Geometry check sheet. Reference: the model listing, model coordinates, mm. Give positions to 0.01 mm unless a question says otherwise; leave off trailing zeros. Order: outer loops, then holes, each group sorted by start corner. A loop starts at its lowest first (then second) coordinate and runs counter-clockwise, first axis right, second up. Notation, with made-up numbers: M 61,-26 L 69,-26 A23 cw 69,-14 Z; hole C -37,3 d4. An arc over 180 degrees is marked long. Answer as a JSON object with one key per item and string values. Group by question number.
from build123d import *

# Parameters (mm, degrees)
F1_DEPTH      = 15
F1_DEPTH_BACK = 15
F2_DEPTH      = 10
F2_DEPTH_BACK = 10
F3_DEPTH      = 5
F3_DEPTH_BACK = 5
F4_R          = 4.99999
F5_T8_DEPTH   = 31.3397459622
F5_S9_R       = 10
F5_T10_DEPTH  = 18
F5_T14_DEPTH  = 31.3397459622
F5_S15_R      = 10
F5_T16_DEPTH  = 18
F5_T20_DEPTH  = 31.3397459622
F5_S21_R      = 10
F5_T22_DEPTH  = 18
F5_T26_DEPTH  = 31.3397459622
F5_S27_R      = 10
F5_T28_DEPTH  = 18


# Not quite as in the source:
# - a fillet or chamfer that OpenCascade refuses, or shapes differently, is made with other operations: its cross-section is extruded or revolved along the edge and cut away or added
# - a fillet or chamfer is up to 0.001 mm smaller than in the source, because OpenCascade refuses the exact size


with BuildPart() as f1:
    # F0 (on Right) → F1 (new body, two sides)
    with BuildSketch(Plane.YZ) as f1_sk:
        with BuildLine():
            Line((-5, 16.4746102661), (5, 16.4746102661))
            ThreePointArc((5, 16.4746102661), (0, 21.4746102661), (-5, 16.4746102661))
        make_face()
        with BuildLine():
            ThreePointArc((-5, 16.4746102661), (0, 11.4746102661), (5, 16.4746102661))
            Line((5, 16.4746102661), (-5, 16.4746102661))
        make_face()
    extrude(amount=F1_DEPTH)
    extrude(f1_sk.sketch, amount=-F1_DEPTH_BACK)

    # F0 (on Right) → F2 (join, two sides)
    with BuildSketch(Plane.YZ) as f2_sk:
        with BuildLine():
            ThreePointArc((-5, 16.4746102661), (0, 21.4746102661), (5, 16.4746102661))
            Line((5, 16.4746102661), (5, 7.8143562283))
            ThreePointArc((5, 7.8143562283), (8.6602540378, 11.4746102661), (10, 16.4746102661))
            ThreePointArc((10, 16.4746102661), (-5, 25.1348643039), (-5, 7.8143562283))
            Line((-5, 7.8143562283), (-5, 16.4746102661))
        make_face()
        with BuildLine():
            Line((5, 7.8143562283), (5, 16.4746102661))
            ThreePointArc((5, 16.4746102661), (0, 11.4746102661), (-5, 16.4746102661))
            Line((-5, 16.4746102661), (-5, 7.8143562283))
            ThreePointArc((-5, 7.8143562283), (0, 6.4746102661), (5, 7.8143562283))
        make_face()
    extrude(amount=F2_DEPTH)
    extrude(f2_sk.sketch, amount=-F2_DEPTH_BACK)

    # F0 (on Right) → F3 (join, two sides)
    with BuildSketch(Plane.YZ) as f3_sk:
        with BuildLine():
            Line((5, 1.4746102661), (5, 7.8143562283))
            ThreePointArc((5, 7.8143562283), (0, 6.4746102661), (-5, 7.8143562283))
            Line((-5, 7.8143562283), (-5, 1.4746102661))
            Line((-5, 1.4746102661), (5, 1.4746102661))
        make_face()
    extrude(amount=F3_DEPTH)
    extrude(f3_sk.sketch, amount=-F3_DEPTH_BACK)

    # F4 (radius 5 in the source; OpenCascade refuses exactly that, so slightly less here)
    f4_edges = [f1.edges().sort_by_distance(p)[0] for p in [
        (15, 5, 16.47461),
        (-15, 5, 16.47461),
    ]]
    fillet(f4_edges, radius=F4_R)

    # F5: fillet of radius 5 on 8 edges, made by hand

    # F5_s1 → F5_t2 (revolve, cut)
    with BuildSketch(Plane.XY.offset(16.4746102661)):
        with BuildLine():
            ThreePointArc((-5, 10), (-8.5355339059, 8.5355339059), (-10, 5))
            Line((-10, 5), (-10, 10))
            Line((-10, 10), (-5, 10))
        make_face()
    revolve(axis=Axis((-10, 0, 16.4746102661), (1, 0, 0)), mode=Mode.SUBTRACT)

    # F5_s3 → F5_t4 (revolve, cut)
    with BuildSketch(Plane.XY.offset(16.4746102661)):
        with BuildLine():
            ThreePointArc((10, 5), (8.5355339059, 8.5355339059), (5, 10))
            Line((5, 10), (10, 10))
            Line((10, 10), (10, 5))
        make_face()
    revolve(axis=Axis((10, 0, 16.4746102661), (1, 0, 0)), mode=Mode.SUBTRACT)


with BuildPart() as f5_tool6:
    # F5_s7 → F5_t8 (new body)
    with BuildSketch(Plane.XY.offset(-11.0253897339)):
        with BuildLine():
            ThreePointArc((-5, 0), (-3.5355339059, 3.5355339059), (0, 5))
            Line((0, 5), (-5, 5))
            Line((-5, 5), (-5, 0))
        make_face()
    extrude(amount=F5_T8_DEPTH)

    # F5_s9 → F5_t10 (cut, symmetric)
    with BuildSketch(Plane.YZ.offset(-2.5)):
        with Locations((0, 16.4746102661)):
            Circle(F5_S9_R)
    extrude(amount=F5_T10_DEPTH, both=True, mode=Mode.SUBTRACT)


with BuildPart() as f1_1:
    add(f1.part)

    # F5_t5: cut F5_tool6
    add(f5_tool6.part, mode=Mode.SUBTRACT)


with BuildPart() as f5_tool12:
    # F5_s13 → F5_t14 (new body)
    with BuildSketch(Plane.XY.offset(-11.0253897339)):
        with BuildLine():
            ThreePointArc((0, 5), (3.5355339059, 3.5355339059), (5, 0))
            Line((5, 0), (5, 5))
            Line((5, 5), (0, 5))
        make_face()
    extrude(amount=F5_T14_DEPTH)

    # F5_s15 → F5_t16 (cut, symmetric)
    with BuildSketch(Plane.YZ.offset(2.5)):
        with Locations((0, 16.4746102661)):
            Circle(F5_S15_R)
    extrude(amount=F5_T16_DEPTH, both=True, mode=Mode.SUBTRACT)


with BuildPart() as f1_2:
    add(f1_1.part)

    # F5_t11: cut F5_tool12
    add(f5_tool12.part, mode=Mode.SUBTRACT)


with BuildPart() as f5_tool18:
    # F5_s19 → F5_t20 (new body)
    with BuildSketch(Plane.XY.offset(20.3143562283)):
        with BuildLine():
            ThreePointArc((0, -5), (3.5355339059, -3.5355339059), (5, 0))
            Line((5, 0), (5, -5))
            Line((5, -5), (0, -5))
        make_face()
    extrude(amount=-F5_T20_DEPTH)

    # F5_s21 → F5_t22 (cut, symmetric)
    with BuildSketch(Plane.YZ.offset(2.5)):
        with Locations((0, 16.4746102661)):
            Circle(F5_S21_R)
    extrude(amount=F5_T22_DEPTH, both=True, mode=Mode.SUBTRACT)


with BuildPart() as f1_3:
    add(f1_2.part)

    # F5_t17: cut F5_tool18
    add(f5_tool18.part, mode=Mode.SUBTRACT)


with BuildPart() as f5_tool24:
    # F5_s25 → F5_t26 (new body)
    with BuildSketch(Plane.XY.offset(20.3143562283)):
        with BuildLine():
            ThreePointArc((0, -5), (-3.5355339059, -3.5355339059), (-5, 0))
            Line((-5, 0), (-5, -5))
            Line((-5, -5), (0, -5))
        make_face()
    extrude(amount=-F5_T26_DEPTH)

    # F5_s27 → F5_t28 (cut, symmetric)
    with BuildSketch(Plane.YZ.offset(-2.5)):
        with Locations((0, 16.4746102661)):
            Circle(F5_S27_R)
    extrude(amount=F5_T28_DEPTH, both=True, mode=Mode.SUBTRACT)


with BuildPart() as f1_4:
    add(f1_3.part)

    # F5_t23: cut F5_tool24
    add(f5_tool24.part, mode=Mode.SUBTRACT)


solid = f1_4.part
1. Depth check by flat-ended pin: pin 1 (4 mm diameter, centred on x = -10, z = 13.5, fed in from -Y); pin 2 (2 mm diameter, centred on y = 2, z = 17, fed in from -X); pin 3 (10 mm diameter, centred on y = -3.5, z = 7, fed in from -X). Enter the tip coordinate at first touch or a pass-through.
2. Cross-section at A-A (x = -1.25). Record the cut outline in (y, z).
3. Thickness scan on line 1 along X through (y, z) = (-5.25, 16.75); line 2 along X through (y, z) = (6.5, 23); line 3 along Y through (x, z) = (-11, 15). Record the ranges inside material, lowest first. Write a range as [from, to].
Report:
{
 "1": {"pin 1": "stops at y = -8.61", "pin 2": "stops at x = -14.88", "pin 3": "stops at x = -10"},
 "2": {"outline": "M -4.84,1.47 L 4.84,1.47 L 4.84,7.72 A10 ccw long -4.84,7.72 Z"},
 "3": {"line 1": "x = [-9.99, 9.99]", "line 2": "x = [-7.7, 7.7]", "line 3": "y = [-4.67, 4.67]"}
}
